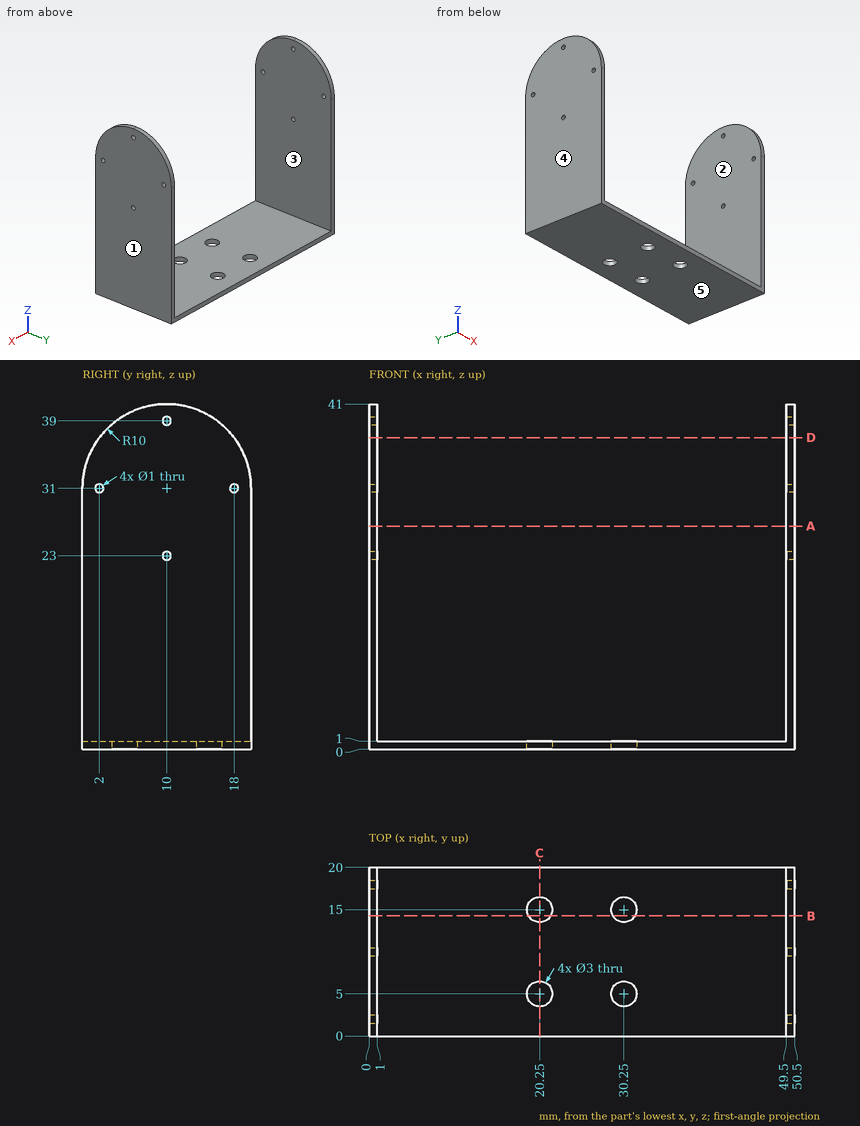
The drawing under review shows one solid part. Ordinate dimensions are in mm from its lowest x, y, z. A direction names the side the tool comes from. Round coordinates to 2 decimals unless told otherwise and drop trailing zeros. Loops run counter-clockwise (first coordinate to the right, second up) from the corner with the lowest first, then second, coordinate; pieces in that order, holes last. Notation, with made-up numbers: (88.25, -26) - (142.25, -26) arc R25 cw to (142.25, 0) - close; hole circle Ø7 at (19.25, 5). An arc over 180 degrees is marked (long way). Use a Markdown table: item, result. Add a question column.
Q1. Insertion check: pin 1 Ø6 at (x, y) = (43.5, 11.5) entering from +Z. The pin has a flat end and moves straight along its axis. Give the tip position at first contact, or say it passes through.
Q2. Add section D-D (z = 37). State the section outline as (x, y) points, plus the area to 3 significant figures.
Q3. Machinability: for the marked faces 1 and 2, which of the approach directions +Z, -Z, +X, -X, +Y, -Y give a long, thin tool a straight path to every point of the face, cutting with its end or side? Answer none if there is none.
Q4. Add section C-C (x = 20.25). State the section outline as (y, z) points.
Q5. Add section A-A (z = 26.5). State the section outline as (x, y) points, plus the area to 3 significant figures.
Q6. The part is to be moulded in two halves that separate along X. For the marked faces 3, 4 and 5, say which applies: pulls with the +X half, pulls with the -X half, needs draft (parallel to the pull), parting line crosses it, or undercut.
Q7. For probe 1 along X at (y, z) = (8.5, 5); probe 2 along Z at (x, y) = (36.5, 16.75); probe 3 along Y at (x, z) = (0.7, 39), list the stretches that pass through material, from the lowest coordinate up.
Q8. Add section B-B (y = 14.25). State the section outline as (x, z) points.
Worked answers:
| question | item | result |
|---|---|---|
| 1 | pin 1 | z = 1 |
| 2 | outline | (0, 2) - (1, 2) - (1, 18) - (0, 18) - close; (49.5, 2) - (50.5, 2) - (50.5, 18) - (49.5, 18) - close |
| 2 | area | 32.0 mm² |
| 3 | face 1 | +Z, -Z, +X, +Y, -Y |
| 3 | face 2 | +Z, +Y, -Y |
| 4 | outline | (0, 0) - (3.5, 0) - (3.5, 1) - (0, 1) - close; (6.5, 0) - (13.5, 0) - (13.5, 1) - (6.5, 1) - close; (16.5, 0) - (20, 0) - (20, 1) - (16.5, 1) - close |
| 5 | outline | (0, 0) - (1, 0) - (1, 20) - (0, 20) - close; (49.5, 0) - (50.5, 0) - (50.5, 20) - (49.5, 20) - close |
| 5 | area | 40.0 mm² |
| 6 | face 3 | undercut |
| 6 | face 4 | pulls with the -X half |
| 6 | face 5 | needs draft |
| 7 | probe 1 | 0 to 1, 49.5 to 50.5 |
| 7 | probe 2 | 0 to 1 |
| 7 | probe 3 | 4 to 9.5, 10.5 to 16 |
| 8 | outline | (0, 0) - (18.95, 0) - (18.95, 1) - (1, 1) - (1, 40.05) - (0, 40.05) - close; (21.55, 0) - (28.95, 0) - (28.95, 1) - (21.55, 1) - close; (31.55, 0) - (50.5, 0) - (50.5, 40.05) - (49.5, 40.05) - (49.5, 1) - (31.55, 1) - close |
